Check sheet for the modelled part. Datum: model origin and axes. Units: mm. A direction names the side the tool comes from. Round coordinates to 2 decimals unless told otherwise and drop trailing zeros. Order: outer loops, then holes, each group sorted by start corner. A loop starts at its lowest first (then second) coordinate and runs counter-clockwise, first axis right, second up.
Autodesk Inventor part; units mm, degrees
ref_plane "YZ Plane" through (0, 0, 0) normal (1, 0, 0) x (0, 1, 0)
ref_plane "XZ Plane" through (0, 0, 0) normal (0, 1, 0) x (-1, 0, 0)
ref_plane "XY Plane" through (0, 0, 0) normal (0, 0, 1) x (1, 0, 0)
sketch "Sketch1" plane through (0, 0, 0) normal (1, 0, 0) x (0, 1, 0)
  circle A0 centre (0, 0) radius 7.5
  line L0 (-31.75, -25.5) -> (-31.75, -20.5)
  line L1 (-31.75, -20.5) -> (-28.75, -20.5)
  line L2 (-28.75, -20.5) -> (-28.75, -10.5)
  line L3 (-28.75, -10.5) -> (-31.75, -10.5)
  line L4 (0, 0) -> (-31.75, 0) construction
  line L5 (-31.75, 20.5) -> (-28.75, 20.5)
  line L6 (-28.75, 20.5) -> (-28.75, 10.5)
  line L7 (-28.75, 10.5) -> (-31.75, 10.5)
  line L8 (-31.75, 25.5) -> (-31.75, 20.5)
  line L9 (-31.75, 10.5) -> (-31.75, -10.5)
  line L10 (-31.75, -20.5) -> (-31.75, -25.5)
  line L11 (20, 25.5) -> (20, 20.5)
  line L12 (20, 20.5) -> (17, 20.5)
  line L13 (17, 20.5) -> (17, 10.5)
  line L14 (17, 10.5) -> (20, 10.5)
  line L15 (20, -20.5) -> (17, -20.5)
  line L16 (17, -20.5) -> (17, -10.5)
  line L17 (17, -10.5) -> (20, -10.5)
  line L18 (20, 25.5) -> (20, 20.5)
  line L19 (20, 10.5) -> (20, -10.5)
  line L20 (20, -20.5) -> (20, -25.5)
  line L21 (20, 25.5) -> (20, 28.5)
  line L22 (-31.75, 28.5) -> (-31.75, 25.5)
  line L23 (-31.75, -25.5) -> (-31.75, -28.5)
  line L24 (20, -28.5) -> (20, -25.5)
  line L25 (-31.75, 28.5) -> (-19.75, 28.5)
  line L26 (-19.75, 28.5) -> (-19.75, 25.5)
  line L27 (-19.75, 25.5) -> (-9.75, 25.5)
  line L28 (-9.75, 25.5) -> (-9.75, 28.5)
  line L29 (-5.875, -28.5) -> (-5.875, 0) construction
  line L30 (8, 28.5) -> (8, 25.5)
  line L31 (8, 25.5) -> (-2, 25.5)
  line L32 (-2, 25.5) -> (-2, 28.5)
  line L33 (-19.75, -28.5) -> (-19.75, -25.5)
  line L34 (-19.75, -25.5) -> (-9.75, -25.5)
  line L35 (-9.75, -25.5) -> (-9.75, -28.5)
  line L36 (8, -25.5) -> (-2, -25.5)
  line L37 (8, -28.5) -> (8, -25.5)
  line L38 (-2, -25.5) -> (-2, -28.5)
  line L39 (-19.75, 28.5) -> (-31.75, 28.5)
  line L40 (20, 28.5) -> (8, 28.5)
  line L41 (-2, 28.5) -> (-9.75, 28.5)
  line L42 (-31.75, -28.5) -> (-19.75, -28.5)
  line L43 (-9.75, -28.5) -> (-2, -28.5)
  line L44 (8, -28.5) -> (20, -28.5)
  line L45 (-31.75, -28.5) -> (-19.75, -28.5)
  line L46 (-9.75, -28.5) -> (-5.875, -28.5)
  line L47 (-28.75, 20.5) -> (-23.5, 20.5) construction
  line L48 (-23.5, 20.5) -> (-23.5, -28.5) construction
  line L49 (-23.5, 0) -> (-23.5, -8) construction
  line L50 (-23.5, -8) -> (-20.5, -8)
  line L51 (-20.5, -8) -> (-20.5, -16)
  line L52 (-20.5, -16) -> (-23.5, -16)
  line L53 (-23.5, -8) -> (-23.5, -16)
  line L54 (-23.5, -20.5) -> (-23.5, 28.5) construction
  line L55 (-23.5, 0) -> (-23.5, 8) construction
  line L56 (-23.5, 8) -> (-20.5, 8)
  line L57 (-20.5, 8) -> (-20.5, 16)
  line L58 (-20.5, 16) -> (-23.5, 16)
  line L59 (-23.5, 8) -> (-23.5, 16)
  line L60 (0, -7.5) -> (0, -9.5) construction
  line L61 (0, -9.5) -> (1.5, -9.5)
  line L62 (1.5, -9.5) -> (1.5, -13.5)
  line L63 (1.5, -13.5) -> (-1.5, -13.5)
  line L64 (-1.5, -13.5) -> (-1.5, -9.5)
  line L65 (-1.5, -9.5) -> (0, -9.5)
  line L66 (0, 9.5) -> (1.5, 9.5)
  line L67 (1.5, 9.5) -> (1.5, 13.5)
  line L68 (1.5, 13.5) -> (-1.5, 13.5)
  line L69 (-1.5, 13.5) -> (-1.5, 9.5)
  line L70 (-1.5, 9.5) -> (0, 9.5)
  line L71 (7.5, 0) -> (9.5, 0) construction
  line L72 (9.5, 0) -> (9.5, -1.5)
  line L73 (9.5, -1.5) -> (13.5, -1.5)
  line L74 (13.5, -1.5) -> (13.5, 1.5)
  line L75 (13.5, 1.5) -> (9.5, 1.5)
  line L76 (9.5, 1.5) -> (9.5, 0)
  line L77 (-7.5, 0) -> (-9.5, 0) construction
  line L78 (-9.5, 0) -> (-9.5, -1.5)
  line L79 (-9.5, -1.5) -> (-13.5, -1.5)
  line L80 (-13.5, -1.5) -> (-13.5, 1.5)
  line L81 (-13.5, 1.5) -> (-9.5, 1.5)
  line L82 (-9.5, 1.5) -> (-9.5, 0)
  dimension "d0" = 15
  dimension "d3" = 51
  dimension "d7" = 5
  dimension "d8" = 3
  dimension "d9" = 10
  dimension "d10" = 3
  dimension "d11" = 51.75
  dimension "d12" = 3
  dimension "d13" = 3
  dimension "d14" = 12
  dimension "d15" = 3
  dimension "d16" = 10
  dimension "d17" = 25.875
  dimension "d18" = 5.25
  dimension "d19" = 8
  dimension "d20" = 3
  dimension "d21" = 8
  dimension "d22" = 2
  dimension "d23" = 1.5
  dimension "d24" = 4
  dimension "d25" = 3
  dimension "d26" = 2
  dimension "d27" = 1.5
  dimension "d28" = 4
  dimension "d29" = 3
extrude "Extrusion1" add sketch "Sketch1" along normal blind 3
sketch "Sketch4" plane through (3, 0, 0) normal (1, 0, 0) x (0, 0, -1)
  line L0 (1.5, 9.5) -> (-1.5, 9.5)
  line L1 (-1.5, 9.5) -> (1.5, 9.5)
  line L2 (1.5, 13.5) -> (1.5, 9.5)
  line L3 (1.5, 9.5) -> (1.5, 13.5)
  line L4 (-1.5, 13.5) -> (1.5, 13.5)
  line L5 (1.5, 13.5) -> (-1.5, 13.5)
  line L6 (-1.5, 9.5) -> (-1.5, 13.5)
  line L7 (-1.5, 13.5) -> (-1.5, 9.5)
  line L8 (-1.5, -9.5) -> (1.5, -9.5)
  line L9 (-1.5, -9.5) -> (1.5, -9.5)
  line L10 (1.5, -9.5) -> (1.5, -13.5)
  line L11 (1.5, -9.5) -> (1.5, -13.5)
  line L12 (1.5, -13.5) -> (-1.5, -13.5)
  line L13 (1.5, -13.5) -> (-1.5, -13.5)
  line L14 (-1.5, -13.5) -> (-1.5, -9.5)
  line L15 (-1.5, -13.5) -> (-1.5, -9.5)
  point P0 (0, 0)
extrude "Extrusion3" add sketch "Sketch4" against normal up to surface (3 mm away)
sketch "Sketch5" plane through (3, 0, 0) normal (1, 0, 0) x (0, 0, -1)
  line L0 (-9.5, -1.5) -> (-13.5, -1.5)
  line L1 (-13.5, -1.5) -> (-13.5, 1.5)
  line L2 (-13.5, 1.5) -> (-9.5, 1.5)
  line L3 (-9.5, 1.5) -> (-9.5, -1.5)
  line L4 (-9.5, -1.5) -> (-13.5, -1.5)
  line L5 (-13.5, -1.5) -> (-13.5, 1.5)
  line L6 (-13.5, -1.5) -> (-13.5, 1.5)
  line L7 (-13.5, 1.5) -> (-9.5, 1.5)
  line L8 (-13.5, 1.5) -> (-9.5, 1.5)
  line L9 (-9.5, 1.5) -> (-9.5, -1.5)
  line L10 (-13.5, -1.5) -> (-9.5, -1.5)
  line L11 (0, 0) -> (0, 8.8912) construction
  line L12 (-8.4853, -10.6066) -> (-10.6066, -8.4853)
  line L13 (-10.6066, -8.4853) -> (-7.7782, -5.6569)
  line L14 (-7.7782, -5.6569) -> (-5.6569, -7.7782)
  line L15 (-8.4853, -10.6066) -> (-5.6569, -7.7782)
  line L16 (8.4853, -10.6066) -> (5.6569, -7.7782)
  line L17 (10.6066, -8.4853) -> (8.4853, -10.6066)
  line L18 (10.6066, -8.4853) -> (7.7782, -5.6569)
  line L19 (5.6569, -7.7782) -> (7.7782, -5.6569)
  line L20 (0, 0) -> (-7.7782, 0) construction
  line L21 (-10.6066, 8.4853) -> (-7.7782, 5.6569)
  line L22 (-8.4853, 10.6066) -> (-10.6066, 8.4853)
  line L23 (-8.4853, 10.6066) -> (-5.6569, 7.7782)
  line L24 (-7.7782, 5.6569) -> (-5.6569, 7.7782)
  line L25 (10.6066, 8.4853) -> (7.7782, 5.6569)
  line L26 (5.6569, 7.7782) -> (7.7782, 5.6569)
  line L27 (8.4853, 10.6066) -> (5.6569, 7.7782)
  line L28 (10.6066, 8.4853) -> (8.4853, 10.6066)
extrude "Extrusion4" cut sketch "Sketch5" against normal up to surface (3 mm away) contours L12 L13 L14 L15 | L16 L19 L18 L17 | L22 L23 L24 L21 | L25 L26 L27 L28
ref_plane "Work Plane1" through (-17.5, 0, 0) normal (1, 0, 0) x (0, 0, -1)
sketch "Sketch6" plane through (-17.5, 0, 0) normal (1, 0, 0) x (0, 0, -1)
  line L0 (8.4853, -10.6066) -> (5.6569, -7.7782)
  line L1 (5.6569, -7.7782) -> (7.7782, -5.6569)
  line L2 (7.7782, -5.6569) -> (10.6066, -8.4853)
  line L3 (10.6066, -8.4853) -> (8.4853, -10.6066)
  line L4 (-5.6569, 7.7782) -> (-7.7782, 5.6569)
  line L5 (-7.7782, 5.6569) -> (-10.6066, 8.4853)
  line L6 (-10.6066, 8.4853) -> (-8.4853, 10.6066)
  line L7 (-8.4853, 10.6066) -> (-5.6569, 7.7782)
  line L8 (10.6066, 8.4853) -> (7.7782, 5.6569)
  line L9 (7.7782, 5.6569) -> (5.6569, 7.7782)
  line L10 (5.6569, 7.7782) -> (8.4853, 10.6066)
  line L11 (8.4853, 10.6066) -> (10.6066, 8.4853)
  line L12 (-7.7782, -5.6569) -> (-5.6569, -7.7782)
  line L13 (-5.6569, -7.7782) -> (-8.4853, -10.6066)
  line L14 (-8.4853, -10.6066) -> (-10.6066, -8.4853)
  line L15 (-10.6066, -8.4853) -> (-7.7782, -5.6569)
  line L16 (-25.5, -2) -> (-28.5, -2)
  line L17 (-28.5, -2) -> (-28.5, -9.75)
  line L18 (-28.5, -9.75) -> (-25.5, -9.75)
  line L19 (-25.5, -9.75) -> (-25.5, -19.75)
  line L20 (-25.5, -19.75) -> (-28.5, -19.75)
  line L21 (-28.5, -19.75) -> (-28.5, -31.75)
  line L22 (-28.5, -31.75) -> (-20.5, -31.75)
  line L23 (-20.5, -31.75) -> (-20.5, -28.75)
  line L24 (-20.5, -28.75) -> (-10.5, -28.75)
  line L25 (-10.5, -28.75) -> (-10.5, -31.75)
  line L26 (-10.5, -31.75) -> (10.5, -31.75)
  line L27 (10.5, -31.75) -> (10.5, -28.75)
  line L28 (10.5, -28.75) -> (20.5, -28.75)
  line L29 (20.5, -28.75) -> (20.5, -31.75)
  line L30 (20.5, -31.75) -> (28.5, -31.75)
  line L31 (28.5, -31.75) -> (28.5, -19.75)
  line L32 (28.5, -19.75) -> (25.5, -19.75)
  line L33 (25.5, -19.75) -> (25.5, -9.75)
  line L34 (25.5, -9.75) -> (28.5, -9.75)
  line L35 (28.5, -9.75) -> (28.5, -2)
  line L36 (28.5, -2) -> (25.5, -2)
  line L37 (25.5, -2) -> (25.5, 8)
  line L38 (25.5, 8) -> (28.5, 8)
  line L39 (28.5, 8) -> (28.5, 20)
  line L40 (28.5, 20) -> (20.5, 20)
  line L41 (20.5, 20) -> (20.5, 17)
  line L42 (20.5, 17) -> (10.5, 17)
  line L43 (10.5, 17) -> (10.5, 20)
  line L44 (10.5, 20) -> (-10.5, 20)
  line L45 (-10.5, 20) -> (-10.5, 17)
  line L46 (-10.5, 17) -> (-20.5, 17)
  line L47 (-20.5, 17) -> (-20.5, 20)
  line L48 (-20.5, 20) -> (-28.5, 20)
  line L49 (-28.5, 20) -> (-28.5, 8)
  line L50 (-28.5, 8) -> (-25.5, 8)
  line L51 (-25.5, 8) -> (-25.5, -2)
  circle A0 centre (0, 0) radius 7.5
  line L52 (16, -20.5) -> (16, -23.5)
  line L53 (16, -23.5) -> (8, -23.5)
  line L54 (8, -23.5) -> (8, -20.5)
  line L55 (8, -20.5) -> (16, -20.5)
  line L56 (-8, -23.5) -> (-16, -23.5)
  line L57 (-16, -23.5) -> (-16, -20.5)
  line L58 (-16, -20.5) -> (-8, -20.5)
  line L59 (-8, -20.5) -> (-8, -23.5)
  line L60 (13.5, 1.5) -> (13.5, -1.5)
  line L61 (13.5, -1.5) -> (9.5, -1.5)
  line L62 (9.5, -1.5) -> (9.5, 1.5)
  line L63 (9.5, 1.5) -> (13.5, 1.5)
  line L64 (-9.5, 1.5) -> (-9.5, -1.5)
  line L65 (-9.5, -1.5) -> (-13.5, -1.5)
  line L66 (-13.5, -1.5) -> (-13.5, 1.5)
  line L67 (-13.5, 1.5) -> (-9.5, 1.5)
  circle A1 centre (0, 0) radius 14.5
  dimension "d40" = 29
sketch "Sketch7" plane through (3, 0, 0) normal (1, 0, 0) x (0, 0, -1)
  line L0 (-13.5, -1.5) -> (-13.5, 1.5)
  line L1 (-9.5, 1.5) -> (-9.5, -1.5)
  line L2 (-13.5, -1.5) -> (-9.5, -1.5)
  line L3 (-9.5, -1.5) -> (-9.5, 1.5)
  line L4 (-9.5, 1.5) -> (-13.5, 1.5)
  line L5 (-13.5, 1.5) -> (-13.5, -1.5)
  line L6 (13.5, -1.5) -> (9.5, -1.5)
  line L7 (13.5, 1.5) -> (13.5, -1.5)
  line L8 (9.5, -1.5) -> (13.5, -1.5)
  line L9 (13.5, -1.5) -> (13.5, 1.5)
  line L10 (13.5, 1.5) -> (9.5, 1.5)
  line L11 (9.5, 1.5) -> (9.5, -1.5)
  point P0 (0, 0)
extrude "Extrusion5" add sketch "Sketch7" against normal up to surface (3 mm away)
sketch "Sketch8" plane through (3, 0, 0) normal (1, 0, 0) x (0, 0, -1)
  line L0 (-8.4853, -10.6066) -> (-5.6569, -7.7782)
  line L1 (-8.4853, -10.6066) -> (-5.6569, -7.7782)
  line L2 (-5.6569, -7.7782) -> (-7.7782, -5.6569)
  line L3 (-5.6569, -7.7782) -> (-7.7782, -5.6569)
  line L4 (-7.7782, -5.6569) -> (-10.6066, -8.4853)
  line L5 (-10.6066, -8.4853) -> (-8.4853, -10.6066)
  line L6 (-10.6066, -8.4853) -> (-8.4853, -10.6066)
  line L7 (1.5, -13.5) -> (1.5, -9.5)
  line L8 (1.5, -9.5) -> (-1.5, -9.5)
  line L9 (-1.5, -9.5) -> (-1.5, -13.5)
  line L10 (-1.5, -13.5) -> (1.5, -13.5)
  point P0 (0, 0)
extrude "Extrusion6" cut sketch "Sketch8" against normal up to surface (3 mm away) contours L10 L9 L8 L7
properties part number "Frontal"
Item 1: Go/stop test with flat-tipped pins: P1, Ø0.9, axis at x = 1, y = -15.5, coming from the +Z side; P2, Ø1.5, axis at x = 1.5, y = 1, coming from the -Z side; P3, Ø12, axis at y = 0, z = 0, coming from the -X side; P4, Ø1.5, axis at x = 1.5, z = 17, coming from the +Y side. Record where each tip stops, or that it passes through.
Answer:
P1: stops at z = 25.5
P2: stops at z = -25.5
P3: passes through
P4: stops at y = 17
Item 2: Access from +Z, -Z, +X, -X, +Y, -Y to the whole of each face (thin tool, end or side, straight path). Record for faces 1 (the flat face through (1, -30, 10.5)), 2 (the flat face through (1, -22, 16)), 3 (the flat face through (1, -15, 25.5)).
Answer:
face 1: +X, -X, -Y
face 2: +X, -X
face 3: +Z, +X, -X
Item 3: Sectioned sample at A-A (z = -4.5). Record the cut outline in (x, y).
Answer:
outline: (0, -31.75) - (3, -31.75) - (3, -6) - (0, -6) - close; (0, 6) - (3, 6) - (3, 20) - (0, 20) - close
Item 4: Scan lines: line 1 along Z through (x, y) = (2.25, -21.5); line 2 along Z through (x, y) = (2.25, 0); line 3 along Z through (x, y) = (2.2, 10.5). Record each from-to range of solid material in increasing order.
Answer:
line 1: z = -28.5 to -16, -8 to 8, 16 to 28.5
line 2: z = -25.5 to -7.5, 7.5 to 25.5
line 3: z = -28.5 to -8.59, -8.38 to 8.38, 8.59 to 28.5
Item 5: Sectioned sample at B-B (y = 0). Record the cut outline in (x, z).
Answer:
outline: (0, -25.5) - (3, -25.5) - (3, -7.5) - (0, -7.5) - close; (0, 7.5) - (3, 7.5) - (3, 25.5) - (0, 25.5) - close
Item 6: Release check for a two-part mould opening along Y. For faces 4 (the flat face through (1, -31.75, 25)), 5 (the flat face through (1.52, -9.56, 9.53)), 6 (the flat face through (3, -6, -6)), 7 (the flat face through (1.52, 9.21, 7.09)) record: released by +Y, released by -Y, zero draft, split by the parting line, or undercut.
Answer:
face 4: released by -Y
face 5: undercut
face 6: zero draft
face 7: undercut
Item 7: Sectioned sample at C-C (x = 2.05). State how many separate pieces and enclosed holes the cut face has, and give its area (3 significant figures).
Answer:
separate pieces: 1
enclosed holes: 8
area: 2,430 mm2
